For this review, take the finished solid that the model builds, in its own axes (mm). Face numbers are marked on the shaded views. A direction names the side the tool comes from. Give positions to 0.01 mm unless a question says otherwise; leave off trailing zeros. Write each loop counter-clockwise with the first axis right and the second up, starting at its lowest first coordinate (ties: lowest second). Pieces come first, ordered by that corner, then holes.
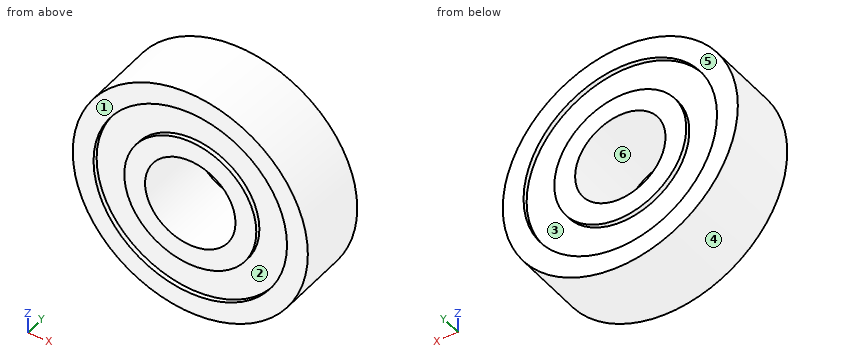
from build123d import *

# Parameters (mm, degrees)
F1_R     = 6.5
F1_R_2   = 5.35
F2_DEPTH = 2
F3_R     = 3.65
F3_R_2   = 2.5
F4_DEPTH = 2
F5_R     = 5.35
F5_R_2   = 3.65
F6_DEPTH = 1.75


with BuildPart() as f2:
    # F1 (on Front) → F2 (new body, symmetric)
    with BuildSketch(Plane.XZ):
        Circle(F1_R)
        Circle(F1_R_2, mode=Mode.SUBTRACT)
    extrude(amount=F2_DEPTH, both=True)



with BuildPart() as f4:
    # F3 (on Front) → F4 (new body, symmetric)
    with BuildSketch(Plane.XZ):
        Circle(F3_R)
        Circle(F3_R_2, mode=Mode.SUBTRACT)
    extrude(amount=F4_DEPTH, both=True)


with BuildPart() as f2_1:
    add(f2.part)

    add(f4.part)  # F6 merges F4
    # F5 (on Front) → F6 (join, symmetric)
    with BuildSketch(Plane.XZ):
        Circle(F5_R)
        Circle(F5_R_2, mode=Mode.SUBTRACT)
    extrude(amount=F6_DEPTH, both=True)


solid = f2_1.part
(1) We need section A-A (z = 0). Write out the cut boundary in (x, y).
(2) The part is to be moulded in two halves that separate along Z. For the marked faces 4, 5 and 6, say which applies: +Z half, -Z half, draft (parallel to the pull), parting line (faces both ways), or undercut.
(3) For L1, parallel to Z at x = 0, y = 1.95; L2, parallel to Y at x = -1.5, z = 4.5; L3, parallel to X at y = 0, z = 0.25, list the stretches that pass through material, from the lowest coordinate up.
(4) We need section B-B (x = 0). Write out the cut boundary in (y, z).
(5) We need section D-D (z = 4.5). Write out the cut boundary in (x, y).
(6) We need section C-C (y = 1.25). Write out the cut boundary in (x, z), and give its area (3 significant figures).
(7) Tool access review of the marked faces 1, 2 and 3: name each direction out of +Z, -Z, +X, -X, +Y, -Y from which nothing blocks a thin tool from reaching the whole face with its end or side.
(8) Clearance check with flat-ended pins moving along their axes: pin 1 Ø1 at (y, z) = (1, 4.5) entering from -X; pin 2 Ø2 at (x, y) = (-2.5, -1.5) entering from +Z. State where each tip first meets the part, or that it passes through.
The answers:
1. outline: (-6.5, -2) - (-5.35, -2) - (-5.35, -1.75) - (-3.65, -1.75) - (-3.65, -2) - (-2.5, -2) - (-2.5, 2) - (-3.65, 2) - (-3.65, 1.75) - (-5.35, 1.75) - (-5.35, 2) - (-6.5, 2) - close; (2.5, -2) - (3.65, -2) - (3.65, -1.75) - (5.35, -1.75) - (5.35, -2) - (6.5, -2) - (6.5, 2) - (5.35, 2) - (5.35, 1.75) - (3.65, 1.75) - (3.65, 2) - (2.5, 2) - close
2. face 4: parting line
2. face 5: draft
2. face 6: undercut
3. L1: z = -6.5 to -5.35, -3.65 to -2.5, 2.5 to 3.65, 5.35 to 6.5
3. L2: y = -1.75 to 1.75
3. L3: x = -6.5 to -2.49, 2.49 to 6.5
4. outline: (-2, -6.5) - (2, -6.5) - (2, -5.35) - (1.75, -5.35) - (1.75, -3.65) - (2, -3.65) - (2, -2.5) - (-2, -2.5) - (-2, -3.65) - (-1.75, -3.65) - (-1.75, -5.35) - (-2, -5.35) - close; (-2, 2.5) - (2, 2.5) - (2, 3.65) - (1.75, 3.65) - (1.75, 5.35) - (2, 5.35) - (2, 6.5) - (-2, 6.5) - (-2, 5.35) - (-1.75, 5.35) - (-1.75, 3.65) - (-2, 3.65) - close
5. outline: (-4.69, -2) - (-2.89, -2) - (-2.89, -1.75) - (2.89, -1.75) - (2.89, -2) - (4.69, -2) - (4.69, 2) - (2.89, 2) - (2.89, 1.75) - (-2.89, 1.75) - (-2.89, 2) - (-4.69, 2) - close
6. outline: circle Ø13 at (0, 0); hole circle Ø5 at (0, 0)
6. area: 113 mm2
7. face 1: +Z, -Z, +X, -X, -Y
7. face 2: -Y
7. face 3: +Y
8. pin 1: stops at x = -5.12
8. pin 2: stops at z = 6.32
